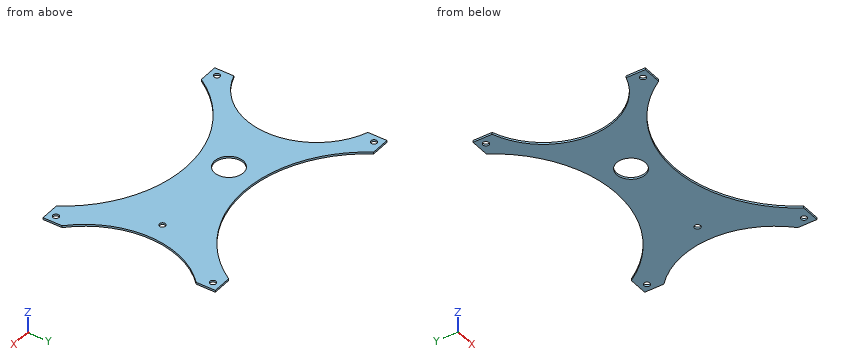
from build123d import *

# Parameters (mm, degrees)
F0_W     = 150
F0_H     = 90
F0_R     = 1.5875
F0_R_2   = 7.5
F1_DEPTH = 1
F2_W     = 21
F2_H     = 90
F3_DEPTH = 1.001
F5_DEPTH = 25


with BuildPart() as f1:
    # F0 (on Top) → F1 (new body)
    with BuildSketch(Plane.XY):
        Rectangle(F0_W, F0_H)
        with Locations((-50, -41)):
            Circle(F0_R, mode=Mode.SUBTRACT)
        with Locations((71, -41)):
            Circle(F0_R, mode=Mode.SUBTRACT)
        with Locations((-50, 41)):
            Circle(F0_R, mode=Mode.SUBTRACT)
        Circle(F0_R_2, mode=Mode.SUBTRACT)
        with Locations((50, 0)):
            Circle(F0_R, mode=Mode.SUBTRACT)
        with Locations((71, 41)):
            Circle(F0_R, mode=Mode.SUBTRACT)
    extrude(amount=F1_DEPTH)

    # F2 (on Top) → F3 (cut, through all)
    with BuildSketch(Plane.XY):
        with Locations((-64.5, 0)):
            Rectangle(F2_W, F2_H)
    extrude(amount=F3_DEPTH, mode=Mode.SUBTRACT)

    # F4 (on Top) → F5 (cut)
    with BuildSketch(Plane.XY):
        with BuildLine():
            ThreePointArc((-44, 45), (10.5, 15), (65, 45))
            Line((65, 45), (-44, 45))
        make_face()
        with BuildLine():
            Line((-54, 35), (-54, -35))
            ThreePointArc((-54, -35), (-29, 0), (-54, 35))
        make_face()
        with BuildLine():
            Line((-44, -45), (65, -45))
            ThreePointArc((65, -45), (10.5, -15), (-44, -45))
        make_face()
        with BuildLine():
            Line((75, -35), (75, 35))
            ThreePointArc((75, 35), (60, 0), (75, -35))
        make_face()
    extrude(amount=F5_DEPTH, mode=Mode.SUBTRACT)


solid = f1.part
Build history of the part. All positions in model axes, mm. Round coordinates to 2 decimals unless told otherwise and drop trailing zeros. Write each loop counter-clockwise with the first axis right and the second up, starting at its lowest first coordinate (ties: lowest second). Pieces come first, ordered by that corner, then holes. Notation, with made-up numbers: M 68,67.5 L 121,67.5 A19 cw 121,85.5 Z; hole C 9,69.25 d7. An arc over 180 degrees is marked long. Answer in a Markdown table with one row per item.
1. Probe L1, parallel to Y at x = -50, z = 0.35; L2, parallel to Y at x = 9.5, z = 0.3; L3, parallel to Y at x = -4.5, z = 0.25. List the from-to ranges inside material, lowest first. Write a range as [from, to].
Geometry check:
| item | result |
|---|---|
| L1 | [-45, -42.59], [-39.41, -33.36], [33.36, 39.41], [42.59, 45] |
| L2 | [-15.01, 15.01] |
| L3 | [-16.77, -6], [6, 16.77] |
2. Saw through at D-D (x = -50). List the corners of the cut face in (y, z), and give its area (3 significant figures).
Geometry check:
| item | result |
|---|---|
| outline | M -45,0 L -42.59,0 L -42.59,1 L -45,1 Z; M -39.41,0 L -33.36,0 L -33.36,1 L -39.41,1 Z; M 33.36,0 L 39.41,0 L 39.41,1 L 33.36,1 Z; M 42.59,0 L 45,0 L 45,1 L 42.59,1 Z |
| area | 16.9 mm2 |
3. Saw through at C-C (y = 6). List the corners of the cut face in (x, z).
Geometry check:
| item | result |
|---|---|
| outline | M -29.49,0 L -4.5,0 L -4.5,1 L -29.49,1 Z; M 4.5,0 L 60.37,0 L 60.37,1 L 4.5,1 Z |
4. Saw through at B-B (z = 0.55). List the corners of the cut face in (x, y) (1 decimal), and give its area (3 significant figures).
Geometry check:
| item | result |
|---|---|
| outline | M -54,-45 L -44,-45 A64.5 cw 65,-45 L 75,-45 L 75,-35 A48.3 cw 75,35 L 75,45 L 65,45 A64.5 cw -44,45 L -54,45 L -54,35 A37 cw -54,-35 Z; hole C -50,-41 d3.2; hole C -50,41 d3.2; hole C 0,0 d15; hole C 50,0 d3.2; hole C 71,-41 d3.2; hole C 71,41 d3.2 |
| area | 4,780 mm2 |
5. Saw through at A-A (x = 50). List the corners of the cut face in (y, z), and give its area (3 significant figures).
Geometry check:
| item | result |
|---|---|
| outline | M -28.51,0 L -1.59,0 L -1.59,1 L -28.51,1 Z; M 1.59,0 L 28.51,0 L 28.51,1 L 1.59,1 Z |
| area | 53.8 mm2 |
